from build123d import *

# Parameters (mm, degrees)
F0_R          = 1.5
F0_W          = 150
F0_H          = 4
F0_H_2        = 31.13
F1_DEPTH      = 2
F2_DEPTH      = 88
F3_R          = 6
F3_R_2        = 1.5
F4_DEPTH      = 3
F4_TAPER      = 45
F5_DEPTH      = 31.131
F5_DEPTH_BACK = 31.131
F6_R          = 2


with BuildPart() as f1:
    # F0 (on Top) → F1 (new body)
    with BuildSketch(Plane.XY):
        Polygon((6.27, 55.26), (-3.73, 55.26), (-16.5067614572, 33.13), (-60.45, 33.13), (-60.45, 28.13), (89.55, 28.13), (89.55, 33.13), (19.0467614572, 33.13), align=None)
        with Locations((1.27, 48.26)):
            Circle(F0_R, mode=Mode.SUBTRACT)
        with Locations((14.55, 26.13)):
            Rectangle(F0_W, F0_H)
        with Locations((14.55, 8.565)):
            Rectangle(F0_W, F0_H_2)
        Circle(F0_R, mode=Mode.SUBTRACT)
        with Locations((82.55, 0)):
            Circle(F0_R, mode=Mode.SUBTRACT)
    extrude(amount=F1_DEPTH)

    # F0 (on Top) → F2 (join)
    with BuildSketch(Plane.XY):
        with Locations((14.55, 26.13)):
            Rectangle(F0_W, F0_H)
    extrude(amount=F2_DEPTH)

    # F3 (on face) → F4 (join)
    with BuildSketch(Plane.XZ.offset(-24.13)):
        with Locations((-49.45, 80)):
            Circle(F3_R)
        with Locations((-49.45, 80)):
            Circle(F3_R_2, mode=Mode.SUBTRACT)
        with Locations((-49.45, 13)):
            Circle(F3_R)
        with Locations((-49.45, 13)):
            Circle(F3_R_2, mode=Mode.SUBTRACT)
        with Locations((78.55, 13)):
            Circle(F3_R)
        with Locations((78.55, 13)):
            Circle(F3_R_2, mode=Mode.SUBTRACT)
        with Locations((78.55, 49)):
            Circle(F3_R)
        with Locations((78.55, 49)):
            Circle(F3_R_2, mode=Mode.SUBTRACT)
        with Locations((-49.45, 80)):
            Circle(F3_R_2)
        with Locations((-49.45, 13)):
            Circle(F3_R_2)
        with Locations((78.55, 13)):
            Circle(F3_R_2)
        with Locations((78.55, 49)):
            Circle(F3_R_2)
    extrude(amount=F4_DEPTH, taper=F4_TAPER)

    # F3 (on face) → F5 (cut, two sides)
    with BuildSketch(Plane.XZ.offset(-24.13)) as f5_sk:
        with Locations((-49.45, 13)):
            Circle(F3_R_2)
        with Locations((78.55, 13)):
            Circle(F3_R_2)
        with Locations((78.55, 49)):
            Circle(F3_R_2)
        with Locations((-49.45, 80)):
            Circle(F3_R_2)
        Polygon((89.55, 88), (-38.45, 88), (4.8512701892, 13), (41.9111145423, 13), (67.55, 57.4078522623), (89.55, 57.4078522623), align=None)
    extrude(amount=F5_DEPTH, mode=Mode.SUBTRACT)
    extrude(f5_sk.sketch, amount=-F5_DEPTH_BACK, mode=Mode.SUBTRACT)

    # F6
    f6_edges = [f1.edges().sort_by_distance(p)[0] for p in [
        (-60.45, 26.13, 88),
        (-38.45, 26.13, 88),
        (4.85127, 26.13, 13),
        (41.911115, 26.13, 13),
        (67.55, 26.13, 57.407852),
        (89.55, 26.13, 57.407852),
        (89.55, -7, 1),
        (89.55, 33.13, 1),
        (19.046761, 33.13, 1),
        (6.27, 55.26, 1),
        (-3.73, 55.26, 1),
        (-16.506761, 33.13, 1),
        (-60.45, 33.13, 1),
        (-60.45, -7, 1),
        (14.55, 24.13, 2),
        (14.55, 28.13, 2),
    ]]
    fillet(f6_edges, radius=F6_R)


solid = f1.part
Read the model definition and answer for the solid it produces. Units are mm, in the model's axes. A direction names the side the tool comes from. Give positions to 0.01 mm unless a question says otherwise; leave off trailing zeros. Write each loop counter-clockwise with the first axis right and the second up, starting at its lowest first coordinate (ties: lowest second). Pieces come first, ordered by that corner, then holes. Notation, with made-up numbers: (-39, -21) - (9, -21) arc R29 cw to (9, 4) - close; hole circle Ø1 at (79.25, 53.5). An arc over 180 degrees is marked (long way). Return JSON: item names as keys, results as strings.
Q1. A cutting plane is placed at B-B, the plane z = 26. Determine the outline of the cut face in (x, y).
Reply:
{"outline": "(-60.45, 24.13) - (-2.65, 24.13) - (-2.65, 28.13) - (-60.45, 28.13) - close; (49.42, 24.13) - (89.55, 24.13) - (89.55, 28.13) - (49.42, 28.13) - close"}
Q2. A cutting plane is placed at D-D, the plane x = 78.55. Determine the outline of the cut face in (y, z).
Reply:
{"outline": "(-7, 0) - (33.13, 0) - (33.13, 2) - (30.13, 2) arc R2 cw to (28.13, 4) - (28.13, 11.5) - (21.13, 11.5) - (21.13, 10) - (24.13, 7) - (24.13, 4) arc R2 cw to (22.13, 2) - (-7, 2) - close; (21.13, 14.5) - (28.13, 14.5) - (28.13, 47.5) - (21.13, 47.5) - (21.13, 46) - (24.13, 43) - (24.13, 19) - (21.13, 16) - close; (21.13, 50.5) - (28.13, 50.5) - (28.13, 57.41) - (24.13, 57.41) - (24.13, 55) - (21.13, 52) - close"}
Q3. A cutting plane is placed at A-A, the plane x = -49.45. Determine the outline of the cut face in (y, z).
Reply:
{"outline": "(-7, 0) - (33.13, 0) - (33.13, 2) - (30.13, 2) arc R2 cw to (28.13, 4) - (28.13, 11.5) - (21.13, 11.5) - (21.13, 10) - (24.13, 7) - (24.13, 4) arc R2 cw to (22.13, 2) - (-7, 2) - close; (21.13, 14.5) - (28.13, 14.5) - (28.13, 78.5) - (21.13, 78.5) - (21.13, 77) - (24.13, 74) - (24.13, 19) - (21.13, 16) - close; (21.13, 81.5) - (28.13, 81.5) - (28.13, 88) - (24.13, 88) - (24.13, 86) - (21.13, 83) - close"}
Q4. For faces 5 (the face through (78, 26, 57.408)), 6 (the face through (83.356, 1.265, 0.986)), 7 (the face through (54.56, 26.1, 34.91)), 8 (the face through (9, 38, 2)), determine the directions among +Z, -Z, +X, -X, +Y, -Y from which every point of the face is accessible in a straight line to the end or side of a thin tool.
Reply:
{"face 5": "+Z, +X, +Y, -Y", "face 6": "+Z, -Z", "face 7": "+Z, +Y, -Y", "face 8": "+Z, +X, -X, +Y"}
Q5. A cutting plane is placed at C-C, the plane x = 26.5. Determine the outline of the cut face in (y, z).
Reply:
{"outline": "(-7, 0) - (33.13, 0) - (33.13, 2) - (30.13, 2) arc R2 cw to (28.13, 4) - (28.13, 13) - (24.13, 13) - (24.13, 4) arc R2 cw to (22.13, 2) - (-7, 2) - close"}
Q6. Consider line 1 along Y through (x, z) = (82.55, 1.3); line 2 along Z through (x, y) = (-49.45, 23.75); line 3 along Y through (x, z) = (0, 1.55). Determine where each line is inside the solid, lowest interval first. Write a range as [from, to].
Reply:
{"line 1": "[-7, -1.5], [1.5, 33.13]", "line 2": "[0, 2.83], [7.38, 11.5], [14.5, 18.62], [74.38, 78.5], [81.5, 85.62]", "line 3": "[-7, -1.5], [1.5, 47.46], [49.06, 55.26]"}
Q7. For a pull along Y with two mould halves and no side action, classify faces 1 (the face through (1.075, 49.747, 0.986)), 2 (the face through (79.356, 24.581, 14.265)), 3 (the face through (12.74, 44.05, 0.99)), 4 (the face through (77, 21.13, 48)) as released by +Y, released by -Y, zero draft, split by the parting line, or undercut.
Reply:
{"face 1": "undercut", "face 2": "zero draft", "face 3": "released by +Y", "face 4": "released by -Y"}
Q8. Given P1, Ø3, axis at x = -48.5, z = 11.5, coming from the -Y side; P2, Ø14.5, axis at x = -6, y = 12, coming from the +Z side; P3, Ø1.6, axis at x = 40, z = 1, coming from the +Y side, each flat-ended and moving along its own axis, determine where each tip first touches the part or whether it passes through.
Reply:
{"P1": "y = 21.13", "P2": "z = 2", "P3": "y = 33.13"}
